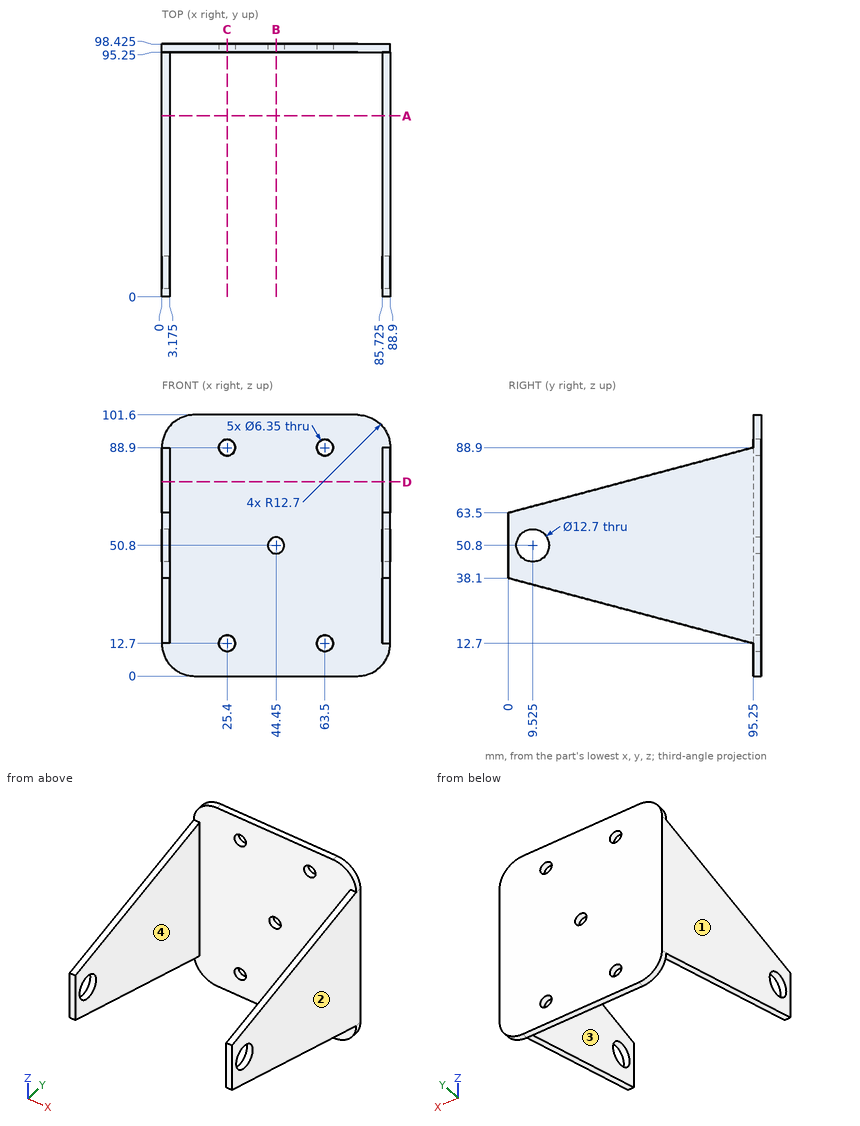
For this review, use the dimensioned drawing (mm, ordinates from the lowest corner) and the shaded views. Coordinates: 2 decimals unless noted, no trailing zeros. Write each loop counter-clockwise with the first axis right and the second up, starting at its lowest first coordinate (ties: lowest second). Pieces come first, ordered by that corner, then holes. Notation, with made-up numbers: (-3.5, -40) - (39.5, -40) arc R11 ccw to (39.5, -31) - close; hole circle Ø2 at (45, 39.5). An arc over 180 degrees is marked (long way). Answer in a Markdown table with one row per item. Add a question column.
Q1. Consider section D-D on z = 75.5. Give the boundary of the cut face in (x, y) (3 decimals), then the cut area to 3 significant figures.
Q2. Consider section A-A on y = 70.5. Give the boundary of the cut face in (x, z) (3 decimals).
Q3. To check wall thickness, follow line 1 along X through (y, z) = (97.4, 88.9) (3 decimals); line 2 along X through (y, z) = (16, 54) (3 decimals); line 3 along Z through (x, y) = (44.45, 96.85) (3 decimals). State the ranges of each line that lie inside material, in increasing order. Write a range as from..to.
Q4. Consider section C-C on x = 25.4. Give the boundary of the cut face in (y, z) (3 decimals), then the cut area to 3 significant figures.
Q5. Consider section B-B on x = 44.45. Give the boundary of the cut face in (y, z) (3 decimals), then the cut area to 3 significant figures.
Q6. Clearance check with flat-ended pins moving along their axes: pin 1 (10 mm diameter, centred on x = 25.4, z = 12.7, fed in from +Y) (3 decimals); pin 2 (4 mm diameter, centred on x = 72, z = 89, fed in from -Y). State where each tip first meets the part, or that it passes through.
Q7. Draft analysis for pull direction X (two halves, no side actions). For the marked faces 1, 2, 3 and 4, state which applies: +X half, -X half, draft (parallel to the pull), parting line (faces both ways), or undercut.
Answers below:
| question | item | result |
|---|---|---|
| 1 | outline | (0, 45) - (3.175, 45) - (3.175, 95.25) - (85.725, 95.25) - (85.725, 45) - (88.9, 45) - (88.9, 98.425) - (0, 98.425) - close |
| 1 | area | 601 mm² |
| 2 | outline | (0, 19.3) - (3.175, 19.3) - (3.175, 82.3) - (0, 82.3) - close; (85.725, 19.3) - (88.9, 19.3) - (88.9, 82.3) - (85.725, 82.3) - close |
| 3 | line 1 | 0..22.225, 28.575..60.325, 66.675..88.9 |
| 3 | line 2 | 0..3.175, 85.725..88.9 |
| 3 | line 3 | 0..47.625, 53.975..101.6 |
| 4 | outline | (95.25, 0) - (98.425, 0) - (98.425, 9.525) - (95.25, 9.525) - close; (95.25, 15.875) - (98.425, 15.875) - (98.425, 85.725) - (95.25, 85.725) - close; (95.25, 92.075) - (98.425, 92.075) - (98.425, 101.6) - (95.25, 101.6) - close |
| 4 | area | 282 mm² |
| 5 | outline | (95.25, 0) - (98.425, 0) - (98.425, 47.625) - (95.25, 47.625) - close; (95.25, 53.975) - (98.425, 53.975) - (98.425, 101.6) - (95.25, 101.6) - close |
| 5 | area | 302 mm² |
| 6 | pin 1 | y = 98.425 |
| 6 | pin 2 | y = 95.25 |
| 7 | face 1 | -X half |
| 7 | face 2 | +X half |
| 7 | face 3 | undercut |
| 7 | face 4 | undercut |
